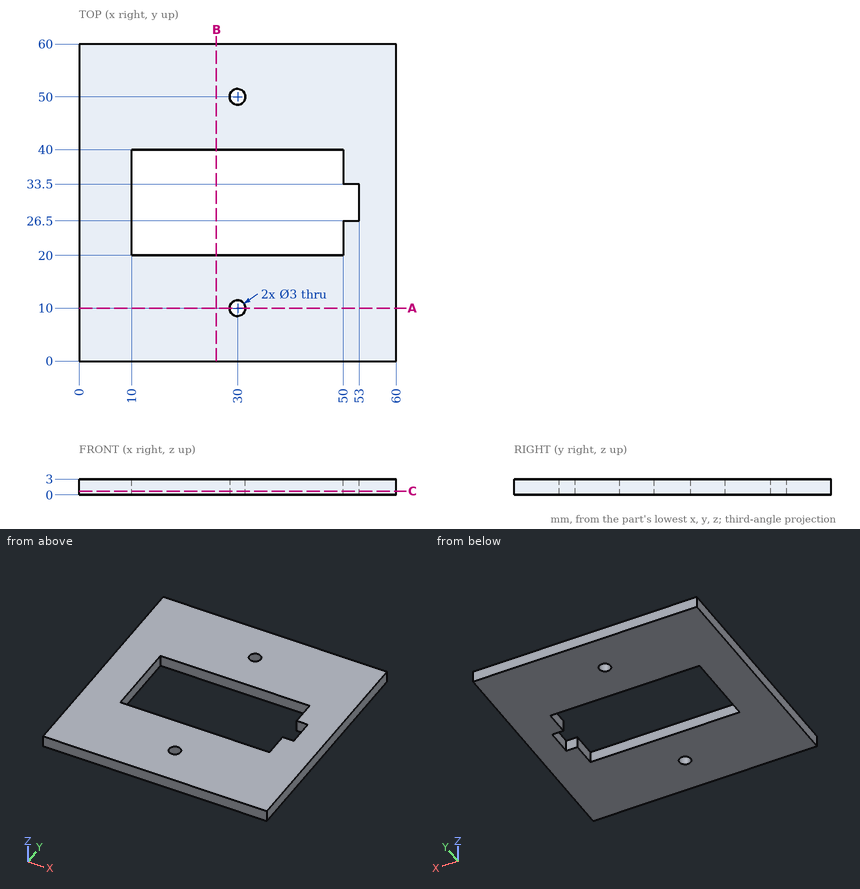
Source: three-view drawing plus pictorial views. Frame: mm from the lowest corner of the part. Give positions to 0.01 mm unless a question says otherwise; leave off trailing zeros. Order: outer loops, then holes, each group sorted by start corner. A loop starts at its lowest first (then second) coordinate and runs counter-clockwise, first axis right, second up. Notation, with made-up numbers: M 85,79 L 118,79 A15 ccw 118,106 Z; hole C 15.5,36 d1. An arc over 180 degrees is marked long. Return JSON: item names as keys, results as strings.
Item 1: Ray query, probe 1 along Y at (x, z) = (30, 1.65); probe 2 along Y at (x, z) = (35, 1.75); probe 3 along X at (y, z) = (50, 1.35). Return the intervals inside material, ascending.
Solutions:
{"probe 1": "0 to 8.5, 11.5 to 20, 40 to 48.5, 51.5 to 60", "probe 2": "0 to 20, 40 to 60", "probe 3": "0 to 28.5, 31.5 to 60"}
Item 2: Cut plane B-B (x = 26). Return loops of the section in (y, z).
Solutions:
{"outline": "M 0,0 L 20,0 L 20,3 L 0,3 Z; M 40,0 L 60,0 L 60,3 L 40,3 Z"}
Item 3: Cut plane A-A (y = 10). Return loops of the section in (x, z), then the cut area to 3 significant figures.
Solutions:
{"outline": "M 0,0 L 28.5,0 L 28.5,3 L 0,3 Z; M 31.5,0 L 60,0 L 60,3 L 31.5,3 Z", "area": "171 mm^2"}
Item 4: Cut plane C-C (z = 0.7). Return loops of the section in (x, y).
Solutions:
{"outline": "M 0,0 L 60,0 L 60,60 L 0,60 Z; hole M 10,20 L 50,20 L 50,26.5 L 53,26.5 L 53,33.5 L 50,33.5 L 50,40 L 10,40 Z; hole C 30,10 d3; hole C 30,50 d3"}
